Geometry: final body of the model. Coordinates: model frame, mm. Face numbers are marked on the shaded views. A direction names the side the tool comes from. Coordinates: 2 decimals unless noted, no trailing zeros. Loops run counter-clockwise (first coordinate to the right, second up) from the corner with the lowest first, then second, coordinate; pieces in that order, holes last. Notation, with made-up numbers: M 6.5,-14.5 L 41.5,-14.5 A26 cw 41.5,6.5 Z; hole C -20.5,12 d2. An arc over 180 degrees is marked long. Write each question's results on one line, items separated by ' | '. Start each with the question number.
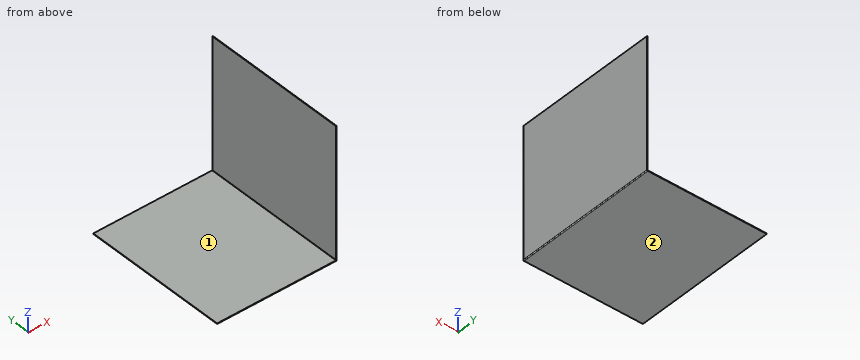
from build123d import *

# Parameters (mm, degrees)
SKETCH1_W                    = 1.5875
SKETCH1_H                    = 400
BASE_FLANGE1_DEPTH           = 330
EDGE_FLANGE1_STRIP_W         = 7.8232
EDGE_FLANGE1_STRIP_H         = 1.5875
EDGE_FLANGE1_STRIP_CUT_DEPTH = 400
EDGE_FLANGE1_DEPTH           = 400


# Sheet-metal steps are written as plain solids
with BuildPart() as part:
    # Sketch1 → Base-Flange1 (new body)
    with BuildSketch(Plane(origin=(0, 0, 0), x_dir=(0, 0, -1), z_dir=(1, 0, 0))):
        with Locations((0.79375, 0)):
            Rectangle(SKETCH1_W, SKETCH1_H)
    extrude(amount=BASE_FLANGE1_DEPTH)

    # Edge-Flange1 strip (across the edge) → Edge-Flange1 strip cut (cut)
    with BuildSketch(Plane(origin=(330, -200, 0), x_dir=(-1, 0, 0), z_dir=(0, 1, 0))):
        with Locations((-1.5875, -0.79375)):
            Rectangle(EDGE_FLANGE1_STRIP_W, EDGE_FLANGE1_STRIP_H)
    extrude(amount=EDGE_FLANGE1_STRIP_CUT_DEPTH, mode=Mode.SUBTRACT)

    # Edge-Flange1 section (across the edge) → Edge-Flange1 (add)
    with BuildSketch(Plane(origin=(330, -200, 0), x_dir=(-1, 0, 0), z_dir=(0, 1, 0))):
        with BuildLine():
            Line((0, 0.7366), (0, 358.4125))
            Line((0, 358.4125), (1.5875, 358.4125))
            Line((1.5875, 358.4125), (1.5875, 0.7366))
            ThreePointArc((1.5875, 0.7366), (1.803245145, 0.215745145), (2.3241, 0))
            Line((2.3241, 0), (2.3241, -1.5875))
            ThreePointArc((2.3241, -1.5875), (0.68071313, -0.90678687), (0, 0.7366))
        make_face()
    extrude(amount=EDGE_FLANGE1_DEPTH)


solid = part.part
Item 1: Ray query, L1, parallel to Z at x = 269, y = -1.5; L2, parallel to X at y = 61.5, z = 235. Return the intervals inside material, ascending. Write a range as [from, to].
Item 2: Contact query for flat-ended pins moving along their axis: P1, Ø3, axis at y = 119, z = 292, coming from the -X side; P2, Ø6, axis at x = 269.5, y = -103.5, coming from the +Z side. Output: stop coordinate, or through.
Item 3: Section A-A, the plane y = -63.5. Return loops of the section in (x, z).
Item 4: Section C-C, the plane z = 122.5. Return loops of the section in (x, y).
Item 5: Set-up query: the marked faces 1 and 2. Return all of +Z, -Z, +X, -X, +Y, -Y with unobstructed straight access to the full face (end or side cutting, diameter ignored); none if empty.
Item 6: Section B-B, the plane x = 155.5. Return loops of the section in (y, z).
Solutions:
1) L1: z = [-1.59, 0] | L2: x = [328.41, 330]
2) P1: stops at x = 328.41 | P2: stops at z = 0
3) outline: M 0,-1.59 L 327.68,-1.59 A2.32 ccw 330,0.74 L 330,358.41 L 328.41,358.41 L 328.41,0.74 A0.74 cw 327.68,0 L 0,0 Z
4) outline: M 328.41,-200 L 330,-200 L 330,200 L 328.41,200 Z
5) face 1: +Z, -X, +Y, -Y | face 2: -Z, +X, -X, +Y, -Y
6) outline: M -200,-1.59 L 200,-1.59 L 200,0 L -200,0 Z
